Geometry check sheet. Reference: the model listing, model coordinates, mm. A direction names the side the tool comes from. Give positions to 0.01 mm unless a question says otherwise; leave off trailing zeros. Write each loop counter-clockwise with the first axis right and the second up, starting at its lowest first coordinate (ties: lowest second). Pieces come first, ordered by that corner, then holes.
(1) Thickness scan on line 1 along Z through (x, y) = (-8, 1); line 2 along X through (y, z) = (-64, 0.5); line 3 along Z through (x, y) = (-7.5, -2). Record the ranges inside material, lowest first.
(2) Tool access check on faces 1 (the cylindrical face through (-6.7, -71, 0.4)), 2 (the flat face through (-15, -74.487, 0)), 3 (the cylindrical face through (-21.546, 32.078, 1.959)). Record the directions out of +Z, -Z, +X, -X, +Y, -Y that give a thin tool (end or side, any length) a straight path to the whole face; none if there is none.
(3) Cross-section at A-A (y = -5). Record the boundary of the cut face in (x, z), and give its area (3 significant figures).
(4) Depth check by flat-ended pin: P1, Ø8, axis at x = -20.5, y = -60, coming from the +Z side; P2, Ø5, axis at x = -8.5, y = -57, coming from the -Z side; P3, Ø6, axis at x = -10.5, y = -15.5, coming from the +Z side. Enter the tip coordinate at first touch or a pass-through.
```python
from build123d import *

# Parameters (mm, degrees)
F3_DEPTH = 5.3848
F4_R     = 0.254
F5_SIZE  = 0.508


# Not quite as in the source:
# - a fillet or chamfer that OpenCascade refuses, or shapes differently, is made with other operations: its cross-section is extruded or revolved along the edge and cut away or added


with BuildPart() as f1:
    # F0 (on Top) → F1 (revolve)
    with BuildSketch(Plane.XY):
        Polygon((-19.1289222062, -69.1020740439), (-15.3252963252, -69.1020740439), (-15.3252963252, 26.1417003232), (-21.4466963252, 26.1417003232), (-22.4372963252, 26.1417003232), (-22.4372963252, 10.0381003232), (-25.5360963252, 1.9012442353), (-25.5360963252, -68.0084118526), (-23.9612963252, -69.5832118526), (-23.9612963252, -72.3429557647), (-25.5360963252, -72.3429557647), (-25.5360963252, -74.4511557647), (-19.1289222062, -74.4511557647), align=None)
        with BuildLine():
            Line((-21.4466963252, 26.1417003232), (-15.3252963252, 26.1417003232))
            Line((-15.3252963252, 26.1417003232), (-15.3252963252, 62.7088442353))
            Line((-15.3252963252, 62.7088442353), (-15.3863094747, 62.7088442353))
            add(Edge.make_bspline(
                [(-15.3863094747, 62.7088442353), (-16.22922346, 62.7838820219), (-16.4167433977, 62.5745207071), (-16.5730696172, 62.435567379)],
                knots=[0, 0, 0, 0, 1.2178176694, 1.2178176694, 1.2178176694, 1.2178176694], degree=3))
            add(Edge.make_bspline(
                [(-16.5730696172, 62.435567379), (-19.0194975585, 56.8844638765), (-20.2809497714, 50.9883202612), (-21.4389152825, 44.2740693688)],
                knots=[0, 0, 0, 0, 18.8020335074, 18.8020335074, 18.8020335074, 18.8020335074], degree=3))
            add(Edge.make_bspline(
                [(-21.8475367874, 37.4826304615), (-21.8703859069, 39.438161999), (-21.8947399408, 42.3613935709), (-21.4389152825, 44.2740693688)],
                knots=[0, 0, 0, 0, 6.8037205974, 6.8037205974, 6.8037205974, 6.8037205974], degree=3))
            Line((-21.8475367874, 37.4826304615), (-21.8475367874, 26.8227737397))
            add(Edge.make_bspline(
                [(-21.8475367874, 26.8227737397), (-21.8473226346, 26.2848939747), (-21.9419963252, 26.1417003232), (-21.4466963252, 26.1417003232)],
                knots=[0, 0, 0, 0, 0.7902746831, 0.7902746831, 0.7902746831, 0.7902746831], degree=3))
        make_face()
    revolve(axis=Axis((-15.3252963252, -24.1547277207, 0), (0, 1, 0)))

    # F2: chamfer of 0.254 on 3 edges, made by hand

    # F2_s1 → F2_t2 (revolve)
    with BuildSketch(Plane.XY):
        Polygon((-22.4372963252, 10.0848293801), (-22.4539271766, 9.9944308884), (-22.4372963252, 10.0381003232), align=None)
    revolve(axis=Axis((-15.3252963252, 10.0381003232, 0), (0, 1, 0)))

    # F2_s3 → F2_t4 (revolve, cut)
    with BuildSketch(Plane.XY):
        Polygon((-19.1289222062, -74.1971557647), (-19.3829222062, -74.4511557647), (-19.1289222062, -74.4511557647), align=None)
    revolve(axis=Axis((-15.3252963252, -74.4511557647, 0), (0, 1, 0)), mode=Mode.SUBTRACT)

    # F2_s5 → F2_t6 (revolve, cut)
    with BuildSketch(Plane.XY):
        Polygon((-22.4372963252, 25.8877003232), (-22.1832963252, 26.1417003232), (-22.4372963252, 26.1417003232), align=None)
    revolve(axis=Axis((-15.3252963252, 26.1417003232, 0), (0, 1, 0)), mode=Mode.SUBTRACT)

    # F3 (add): a face of the model
    f3_faces = [f1.faces().sort_by_distance(p)[0] for p in [
        (-15.3252963252, -69.1020740439, 0),
    ]]
    extrude(f3_faces, amount=F3_DEPTH)

    # F4
    f4_edges = [f1.edges().sort_by_distance(p)[0] for p in [
        (-11.52167, -74.486874, 0),
    ]]
    fillet(f4_edges, radius=F4_R)

    # F5
    f5_edges = [f1.edges().sort_by_distance(p)[0] for p in [
        (-5.114496, -74.451156, 0),
    ]]
    chamfer(f5_edges, length=F5_SIZE)


solid = f1.part
```
Reply:
1. line 1: z = -7.11 to 7.11
1. line 2: x = -25.52 to -5.13
1. line 3: z = -6.56 to 6.56
2. face 1: none
2. face 2: +Z, -Z, +X, -X, -Y
2. face 3: +Y
3. outline: circle Ø20.42 at (-15.33, 0)
3. area: 328 mm2
4. P1: stops at z = 10.14
4. P2: stops at z = -9.25
4. P3: stops at z = 10.05
